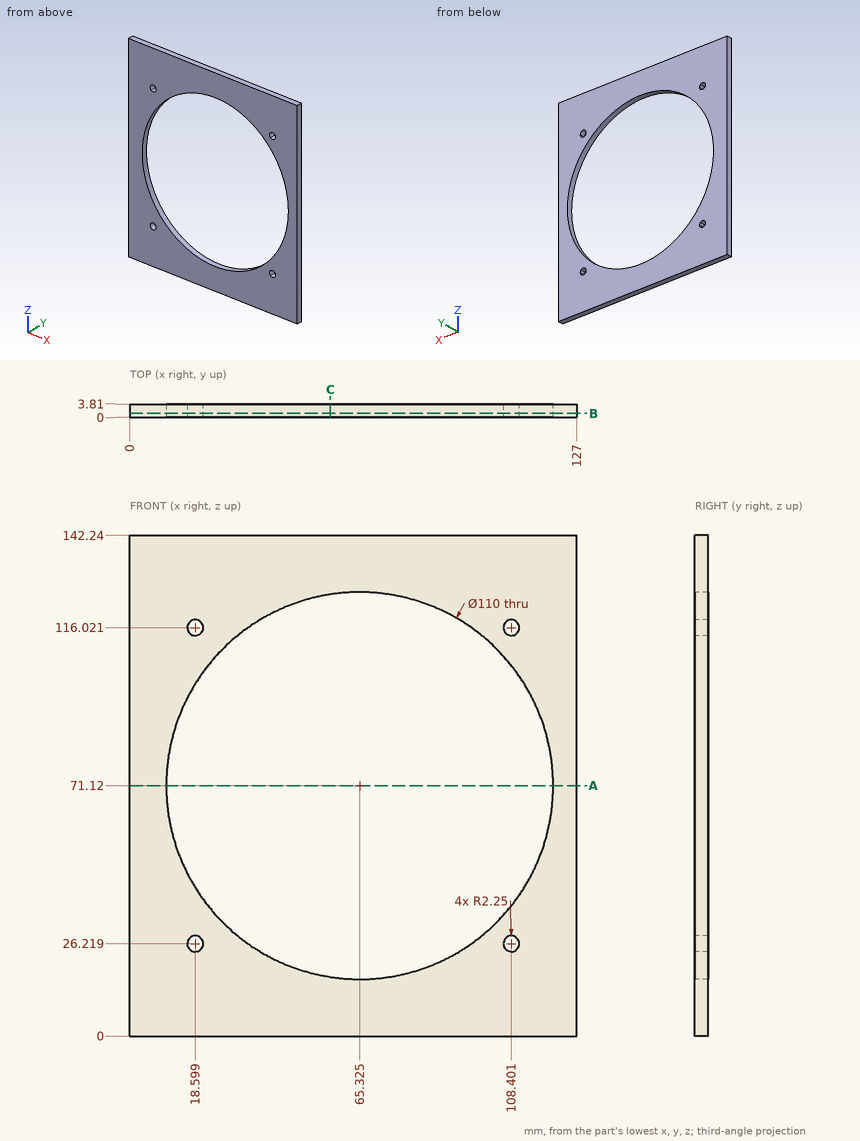
Job drawing, mm, ordinate dimensions from the low corner. One solid piece. Give positions to 0.01 mm unless a question says otherwise; leave off trailing zeros. Loops run counter-clockwise (first coordinate to the right, second up) from the corner with the lowest first, then second, coordinate; pieces in that order, holes last. Notation, with made-up numbers: M -36.75,71 L 16.25,71 A27 cw 16.25,104 Z; hole C -25.5,41 d11. An arc over 180 degrees is marked long. Put each result on its own line as item: value. Start each with the question number.
1) Saw through at B-B (y = 1.15). State how many separate pieces and enclosed holes the cut face has, then the cut area to 3 significant figures.
2) Saw through at C-C (x = 57). List the corners of the cut face in (y, z), then the cut area to 3 significant figures.
3) Probe probe 1 along Z at (x, y) = (108, 2.5) (1 decimal); probe 2 along X at (y, z) = (3.1, 71) (1 decimal); probe 3 along Z at (x, y) = (53, 0.7). List the from-to ranges inside material, lowest first.
4) Saw through at A-A (z = 71.12). List the corners of the cut face in (x, y) (1 decimal).
Numbers:
1. separate pieces: 1
1. enclosed holes: 5
1. area: 8,500 mm^2
2. outline: M 0,0 L 3.81,0 L 3.81,16.75 L 0,16.75 Z; M 0,125.49 L 3.81,125.49 L 3.81,142.24 L 0,142.24 Z
2. area: 128 mm^2
3. probe 1: 0 to 24, 28.4 to 36.4, 105.8 to 113.8, 118.2 to 142.2
3. probe 2: 0 to 10.3, 120.3 to 127
3. probe 3: 0 to 17.52, 124.72 to 142.24
4. outline: M 0,0 L 10.3,0 L 10.3,3.8 L 0,3.8 Z; M 120.3,0 L 127,0 L 127,3.8 L 120.3,3.8 Z
